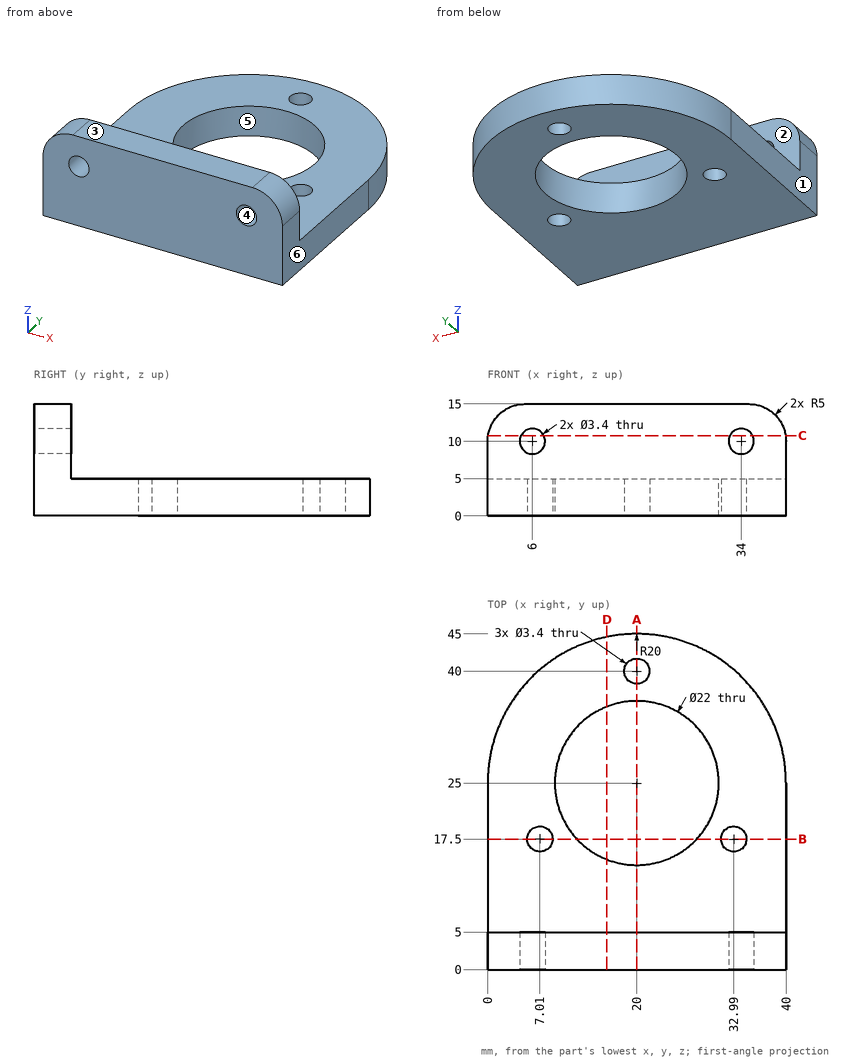
Print and shaded views of the part. All mm, measured from the part's lowest x, y and z. A direction names the side the tool comes from. Give positions to 0.01 mm unless a question says otherwise; leave off trailing zeros. Order: outer loops, then holes, each group sorted by start corner. A loop starts at its lowest first (then second) coordinate and runs counter-clockwise, first axis right, second up. Notation, with made-up numbers: M 74,55 L 128,55 A29 ccw 128,92 Z; hole C 53,34.25 d2. An arc over 180 degrees is marked long. Use one line per item in the form item = value.
Q1. Pull direction X, two halves, no side cores. Call the marked faces 3, 4, 5 and 6: released by +X, released by -X, zero draft, split by the parting line, or undercut.
Conclusion:
face_3 = zero draft
face_4 = undercut
face_5 = undercut
face_6 = released by +X
Q2. Slice it at D-D, the plane x = 16. Write the cut outline in (y, z).
Conclusion:
outline = M 0,0 L 14.75,0 L 14.75,5 L 5,5 L 5,15 L 0,15 Z; M 35.25,0 L 44.6,0 L 44.6,5 L 35.25,5 Z
Q3. Slice it at C-C, the plane z = 10.75. Write the cut outline in (x, y) (1 decimal), and give its area (3 significant figures).
Conclusion:
outline = M 0.1,0 L 4.5,0 L 4.5,5 L 0.1,5 Z; M 7.5,0 L 32.5,0 L 32.5,5 L 7.5,5 Z; M 35.5,0 L 39.9,0 L 39.9,5 L 35.5,5 Z
area = 169 mm2
Q4. Which spindle directions (+Z, -Z, +X, -X, +Y, -Y) get a long thin tool onto all of the face, cutting with end or side? Do the marked faces 1 and 2. Say none if no direction does.
Conclusion:
face_1 = +Z, -Z, -X, +Y, -Y
face_2 = +Z, +X, -X, +Y
Q5. Pin check, flat tips, straight feed: P1, Ø8, axis at x = 17.5, z = 11.5, coming from the +Y side; P2, Ø5.5, axis at x = 32.99, y = 17.5, coming from the +Z side; P3, Ø3, axis at x = 14, z = 4.5, coming from the +Y side. Stop position of each tip, or through.
Conclusion:
P1 = 5
P2 = 5
P3 = 44.49
Q6. Slice it at A-A, the plane x = 20. Write the cut outline in (y, z).
Conclusion:
outline = M 0,0 L 14,0 L 14,5 L 5,5 L 5,15 L 0,15 Z; M 36,0 L 38.3,0 L 38.3,5 L 36,5 Z; M 41.7,0 L 45,0 L 45,5 L 41.7,5 Z
Q7. Wall check: probe 1 along X at (y, z) = (3.6, 10); probe 2 along Y at (x, z) = (20, 1.5); probe 3 along Y at (x, z) = (9, 6.5). Give the ranges that are in metal, low to high.
Conclusion:
probe_1 = 0 to 4.3, 7.7 to 32.3, 35.7 to 40
probe_2 = 0 to 14, 36 to 38.3, 41.7 to 45
probe_3 = 0 to 5
Q8. Slice it at B-B, the plane y = 17.5. Write the cut outline in (x, z).
Conclusion:
outline = M 0,0 L 5.31,0 L 5.31,5 L 0,5 Z; M 8.71,0 L 11.95,0 L 11.95,5 L 8.71,5 Z; M 28.05,0 L 31.29,0 L 31.29,5 L 28.05,5 Z; M 34.69,0 L 40,0 L 40,5 L 34.69,5 Z
